```python
from build123d import *

# Parameters (mm, degrees)
F1_DEPTH = 50
F2_W     = 30
F2_H     = 91
F2_W_2   = 22
F3_DEPTH = 37
F4_W     = 24
F4_H     = 12.44826
F4_R     = 3.5
F4_W_2   = 24.552317
F4_H_2   = 31
F5_DEPTH = 30
F6_W     = 12
F6_H     = 30
F6_R     = 2
F7_DEPTH = 3.001


with BuildPart() as f1:
    # F0 (on Right) → F1 (new body, symmetric)
    with BuildSketch(Plane.YZ):
        Polygon((0, 40), (-35.697561, 40), (-95, 0), (0, 0), align=None)
    extrude(amount=F1_DEPTH, both=True)

    # F2 (on face) → F3 (cut)
    with BuildSketch(Plane.XY.offset(40)):
        with Locations((-30, -49.5)):
            Rectangle(F2_W, F2_H)
        with Locations((30, -49.5)):
            Rectangle(F2_W, F2_H)
        with Locations((0, -49.5)):
            Rectangle(F2_W_2, F2_H)
    extrude(amount=-F3_DEPTH, mode=Mode.SUBTRACT)

    # F4 (on face) → F5 (cut, through all)
    with BuildSketch(Plane.YZ.offset(15)):
        with Locations((-48.552317, 9.22413)):
            Rectangle(F4_W, F4_H)
        with Locations((-40.052317, 30)):
            Circle(F4_R)
        with Locations((-16.276159, 18.5)):
            Rectangle(F4_W_2, F4_H_2)
    extrude(amount=-F5_DEPTH, mode=Mode.SUBTRACT)

    # F6 (on face) → F7 (cut, through all)
    with BuildSketch(Plane.XY.offset(3)):
        with Locations((-39, -24.347831)):
            Rectangle(F6_W, F6_H)
        with Locations((39, -24.347831)):
            Rectangle(F6_W, F6_H)
        with Locations((-26.107078, -10.847831)):
            Circle(F6_R)
        with Locations((-26.107078, -37.847831)):
            Circle(F6_R)
        with Locations((26.107078, -10.847831)):
            Circle(F6_R)
        with Locations((26.107078, -37.847831)):
            Circle(F6_R)
    extrude(amount=-F7_DEPTH, mode=Mode.SUBTRACT)


solid = f1.part
```
CAD build for the part. Positions are in the model's coordinates, mm. A direction names the side the tool comes from. Give positions to 0.01 mm unless a question says otherwise; leave off trailing zeros. Write each loop counter-clockwise with the first axis right and the second up, starting at its lowest first coordinate (ties: lowest second). Pieces come first, ordered by that corner, then holes. Notation, with made-up numbers: M -6.5,46.25 L 11.5,46.25 A22 ccw 11.5,67.25 Z; hole C 74,52.25 d7. An arc over 180 degrees is marked long. Return JSON: item names as keys, results as strings. Group by question number.
(1) Mould opens along Z. For faces 1 (the face through (-13, -49, 15.448)), 2 (the face through (0, -4, 22)), 3 (the face through (13, -60.552, 9)), 4 (the face through (1, -48, 0)) say: pulls with the +Z half, pulls with the -Z half, needs draft (parallel to the pull), parting line crosses it, or undercut.
(2) Band-saw the part on B-B (z = 22.5). Give the cut face in (x, y), and give its area (3 significant figures).
(3) Band-saw the part on A-A (y = -23.5). Give the cut face in (x, z), and give its area (3 significant figures).
(4) Flat gauge pins, fed straight in: pin 1 Ø2.5 at (x, z) = (39, 1.5) entering from -Y; pin 2 Ø1 at (x, y) = (-4, -16.5) entering from +Z; pin 3 Ø3.5 at (x, z) = (-40.5, 1.5) entering from -Y. Where does each tip first touch, or does it go through?
(5) Band-saw the part on C-C (z = 9.5). Give the cut face in (x, y), and give its area (3 significant figures).
(6) Band-saw the part on D-D (x = -5). Give the cut face in (y, z), and give its area (3 significant figures).
(7) 3-axis set-ups, long thin cutter, end or side, ignore diameter. For faces 5 (the face through (-33, -25, 2)), 6 (the face through (-14.58, -71.8, 15.65)), 7 (the face through (-15, -38, 22)), 8 (the face through (13, -49, 15.448)), 9 (the face through (50, -38, 16)): which of +Z, -Z, +X, -X, +Y, -Y reach the whole face in a straight line?
(8) Drill centre lines: L1, parallel to X at y = -47, z = 26.5; L2, parallel to X at y = -17, z = 9; L3, parallel to Y at x = -0.5, z = 35. Where is each one in solid material? Low to high. Write a range as [from, to].
Entries:
{
 "1": {"face 1": "undercut", "face 2": "needs draft", "face 3": "undercut", "face 4": "pulls with the -Z half"},
 "2": {"outline": "M -50,-61.64 L -45,-61.64 L -45,-4 L 45,-4 L 45,-61.64 L 50,-61.64 L 50,0 L -50,0 Z; M -15,-61.64 L -11,-61.64 L -11,-28.55 L -15,-28.55 Z; M 11,-61.64 L 15,-61.64 L 15,-28.55 L 11,-28.55 Z", "area": "1,240 mm^2"},
 "3": {"outline": "M -50,0 L -45,0 L -45,40 L -50,40 Z; M -33,0 L 33,0 L 33,3 L -33,3 Z; M -15,34 L -11,34 L -11,40 L -15,40 Z; M 11,34 L 15,34 L 15,40 L 11,40 Z; M 45,0 L 50,0 L 50,40 L 45,40 Z", "area": "646 mm^2"},
 "4": {"pin 1": "stops at y = -94.63", "pin 2": "stops at z = 3", "pin 3": "stops at y = -95"},
 "5": {"outline": "M -50,-80.92 L -45,-80.92 L -45,-4 L 45,-4 L 45,-80.92 L 50,-80.92 L 50,0 L -50,0 Z; M -15,-80.92 L -11,-80.92 L -11,-60.55 L -15,-60.55 Z; M -15,-36.55 L -11,-36.55 L -11,-28.55 L -15,-28.55 Z; M 11,-80.92 L 15,-80.92 L 15,-60.55 L 11,-60.55 Z; M 11,-36.55 L 15,-36.55 L 15,-28.55 L 11,-28.55 Z", "area": "1,400 mm^2"},
 "6": {"outline": "M -95,0 L 0,0 L 0,40 L -4,40 L -4,3 L -90.55,3 Z", "area": "426 mm^2"},
 "7": {"face 5": "+Z, -Z", "face 6": "+Z, +X, -X, -Y", "face 7": "+Z, -Y", "face 8": "none", "face 9": "+Z, -Z, +X, +Y, -Y"},
 "8": {"L1": "x = [-50, -45], [-15, -11], [11, 15], [45, 50]", "L2": "x = [-50, -45], [45, 50]", "L3": "y = [-4, 0]"}
}
